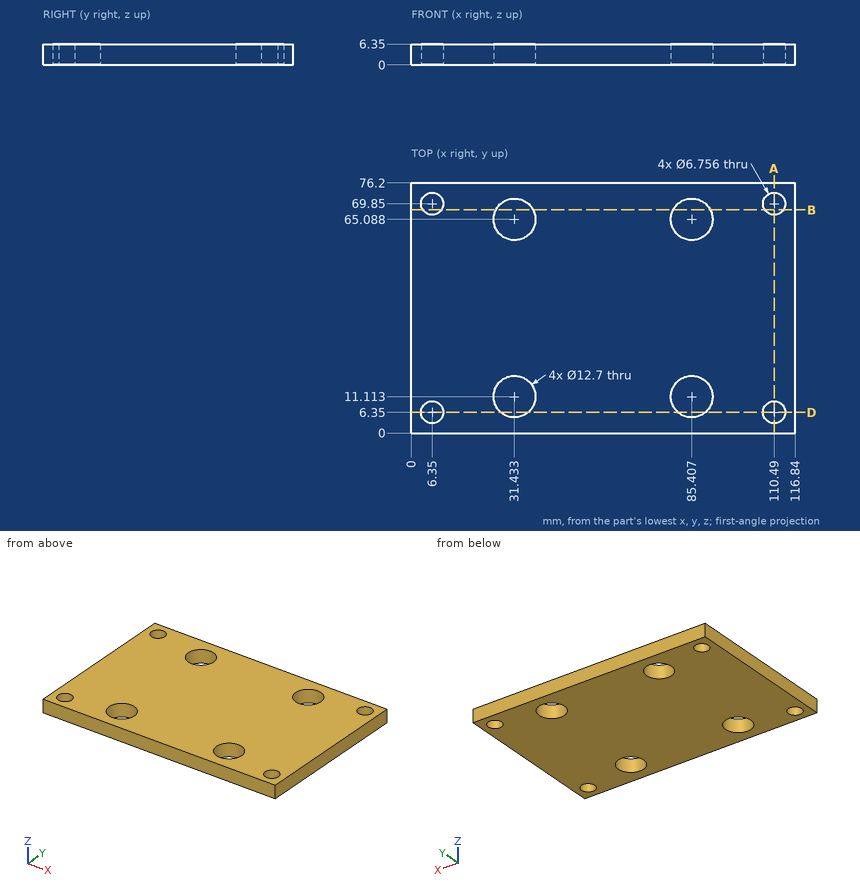
Answer from the drawing. Dimensions are ordinates in mm from the lowest x, y and z of the part. Give positions to 0.01 mm unless a question says otherwise; leave off trailing zeros. Loops run counter-clockwise (first coordinate to the right, second up) from the corner with the lowest first, then second, coordinate; pieces in that order, holes last. Notation, with made-up numbers: (39, -26) -> (58, -26) arc R37 cw to (58, 13) -> close; hole circle Ø4 at (80, 5.25). An arc over 180 degrees is marked (long way). Use a Markdown table: item, result.
Q1. Section A-A, the plane x = 110.49 is taken. Determine the outline of the cut face in (y, z).
Solved:
| item | result |
|---|---|
| outline | (0, 0) -> (2.97, 0) -> (2.97, 6.35) -> (0, 6.35) -> close; (9.73, 0) -> (66.47, 0) -> (66.47, 6.35) -> (9.73, 6.35) -> close; (73.23, 0) -> (76.2, 0) -> (76.2, 6.35) -> (73.23, 6.35) -> close |
Q2. This flat-tipped pin is pushed along its axis until it touches: pin 1 (11 mm diameter, centred on x = 110.49, y = 6.35, fed in from +Z). Where does it stop, or does it pass through?
Solved:
| item | result |
|---|---|
| pin 1 | stops at z = 6.35 |
Q3. Section B-B, the plane y = 68 is taken. Count the separate pieces of the cut face and the enclosed holes in it, then the cut area to 3 significant figures.
Solved:
| item | result |
|---|---|
| separate pieces | 5 |
| enclosed holes | 0 |
| area | 527 mm^2 |
Q4. Section D-D, the plane y = 6.35 is taken. Determine the outline of the cut face in (x, z).
Solved:
| item | result |
|---|---|
| outline | (0, 0) -> (2.97, 0) -> (2.97, 6.35) -> (0, 6.35) -> close; (9.73, 0) -> (27.23, 0) -> (27.23, 6.35) -> (9.73, 6.35) -> close; (35.63, 0) -> (81.21, 0) -> (81.21, 6.35) -> (35.63, 6.35) -> close; (89.61, 0) -> (107.11, 0) -> (107.11, 6.35) -> (89.61, 6.35) -> close; (113.87, 0) -> (116.84, 0) -> (116.84, 6.35) -> (113.87, 6.35) -> close |
Q5. Find the intervals of material crossed by line 1 along Y through (x, z) = (110.49, 5); line 2 along X through (y, z) = (60, 4) (1 decimal); line 3 along Y through (x, z) = (9, 6) (1 decimal), in increasing order.
Solved:
| item | result |
|---|---|
| line 1 | y = 0 to 2.97, 9.73 to 66.47, 73.23 to 76.2 |
| line 2 | x = 0 to 27.6, 35.2 to 81.6, 89.2 to 116.8 |
| line 3 | y = 0 to 4.3, 8.4 to 67.8, 71.9 to 76.2 |
